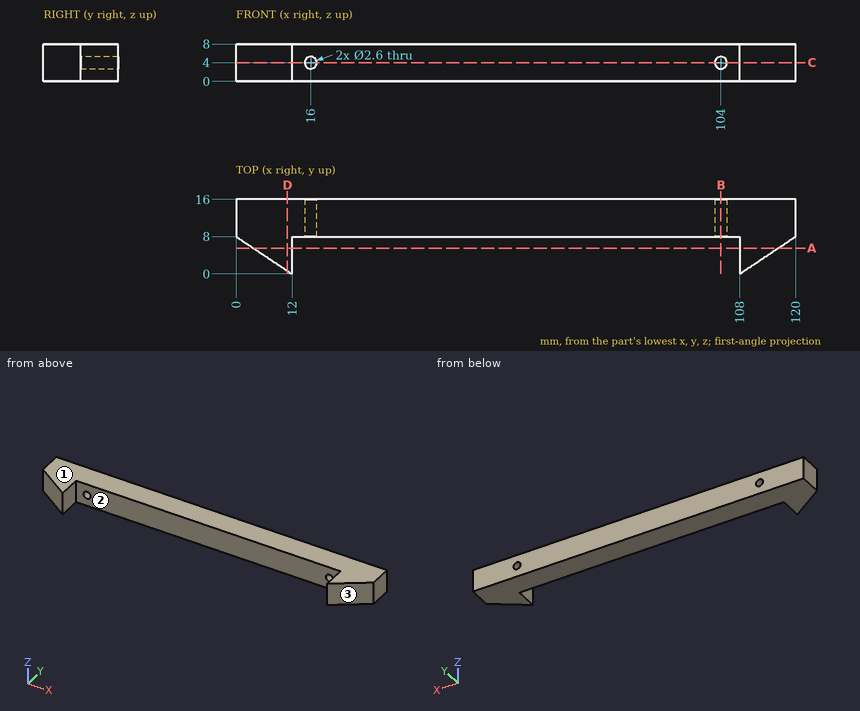
Drawing for the job (mm, zero at the part's lowest x, y, z). Round coordinates to 2 decimals unless told otherwise and drop trailing zeros. Order: outer loops, then holes, each group sorted by start corner. A loop starts at its lowest first (then second) coordinate and runs counter-clockwise, first axis right, second up. Notation, with made-up numbers: (-11, 22.25) -> (3, 22.25) arc R22 cw to (3, 56.25) -> close; hole circle Ø3 at (83.25, -27.75). An arc over 180 degrees is marked (long way). Put each result on its own line as item: value.
Q1. Pin check, flat tips, straight feed: pin 1 Ø4 at (x, z) = (54.5, 2.5) entering from -Y; pin 2 Ø1.6 at (x, z) = (16, 4) entering from +Y; pin 3 Ø3 at (x, z) = (107.5, 3.5) entering from -Y; pin 4 Ø2.5 at (y, z) = (2.5, 2.5) entering from -X (3 decimals). Stop position of each tip, or through.
From the geometry:
pin 1: stops at y = 8
pin 2: passes through
pin 3: stops at y = 0
pin 4: stops at x = 6.375
Q2. Wall check: line 1 (Z direction, x = 104, y = 13); line 2 (Y direction, x = 65.5, z = 6); line 3 (X direction, y = 13, z = 3). Give the ranges that are in metal, low to high. Write a range as [from, to].
From the geometry:
line 1: z = [0, 2.7], [5.3, 8]
line 2: y = [8, 16]
line 3: x = [0, 15.17], [16.83, 103.17], [104.83, 120]
Q3. Band-saw the part on D-D (x = 11). Give the cut face in (y, z), and give its area (3 significant figures).
From the geometry:
outline: (0.67, 0) -> (16, 0) -> (16, 8) -> (0.67, 8) -> close
area: 123 mm2
Q4. Band-saw the part on A-A (y = 5.5). Give the cut face in (x, z), and give its area (3 significant figures).
From the geometry:
outline: (3.75, 0) -> (12, 0) -> (12, 8) -> (3.75, 8) -> close; (108, 0) -> (116.25, 0) -> (116.25, 8) -> (108, 8) -> close
area: 132 mm2
Q5. Pull direction X, two halves, no side cores. Call the marked faces 1, 2 and 3: pulls with the +X half, pulls with the -X half, needs draft (parallel to the pull), parting line crosses it, or undercut.
From the geometry:
face 1: needs draft
face 2: undercut
face 3: pulls with the +X half
Q6. Band-saw the part on B-B (x = 104). Give the cut face in (y, z).
From the geometry:
outline: (8, 0) -> (16, 0) -> (16, 2.7) -> (8, 2.7) -> close; (8, 5.3) -> (16, 5.3) -> (16, 8) -> (8, 8) -> close
Q7. Band-saw the part on C-C (z = 4). Give the cut face in (x, y), and give its area (3 significant figures).
From the geometry:
outline: (0, 8) -> (12, 0) -> (12, 8) -> (14.7, 8) -> (14.7, 16) -> (0, 16) -> close; (17.3, 8) -> (102.7, 8) -> (102.7, 16) -> (17.3, 16) -> close; (105.3, 8) -> (108, 8) -> (108, 0) -> (120, 8) -> (120, 16) -> (105.3, 16) -> close
area: 1,010 mm2
